Check sheet for the modelled part. Datum: model origin and axes. Units: mm. A direction names the side the tool comes from. Coordinates: 2 decimals unless noted, no trailing zeros. Loops run counter-clockwise (first coordinate to the right, second up) from the corner with the lowest first, then second, coordinate; pieces in that order, holes last. Notation, with made-up numbers: (68.25, 36) -> (121.25, 36) arc R26 ccw to (121.25, 61) -> close; hole circle Ø8 at (4.5, -11). An arc over 180 degrees is marked (long way). Use one line per item in the form item = value.
from build123d import *

# Parameters (mm, degrees)
F0_R     = 10
F1_DEPTH = 1.5
F2_R     = 5
F3_DEPTH = 1
F4_R     = 4
F5_DEPTH = 3
F6_R     = 0.75


with BuildPart() as f1:
    # F0 (on Top) → F1 (new body)
    with BuildSketch(Plane.XY):
        Circle(F0_R)
    extrude(amount=F1_DEPTH)

    # F2 (on face) → F3 (join)
    with BuildSketch(Plane.XY.offset(1.5)):
        Circle(F2_R)
    extrude(amount=F3_DEPTH)

    # F4 (on face) → F5 (join)
    with BuildSketch(Plane.XY.offset(2.5)):
        Circle(F4_R)
    extrude(amount=F5_DEPTH)

    # F6
    f6_edges = [f1.edges().sort_by_distance(p)[0] for p in [
        (-10, 0, 0),
    ]]
    fillet(f6_edges, radius=F6_R)


solid = f1.part
(1) Tool access check on faces 1 (the cylindrical face through (-2.17, -9.76, 1.12)), 2 (the flat face through (-5, -2, 1.5)). Record the directions out of +Z, -Z, +X, -X, +Y, -Y that give a thin tool (end or side, any length) a straight path to the whole face; none if there is none.
Established:
face_1 = +Z, -Z
face_2 = +Z
(2) Section check C-C, the plane z = 1.15. Record the boundary of the cut face in (x, y).
Established:
outline = circle Ø20 at (0, 0)
(3) Section check D-D, the plane z = 2.9. Record the boundary of the cut face in (x, y).
Established:
outline = circle Ø8 at (0, 0)
(4) Section check A-A, the plane x = 0. Record the boundary of the cut face in (y, z).
Established:
outline = (-10, 0.75) arc R0.75 ccw to (-9.25, 0) -> (9.25, 0) arc R0.75 ccw to (10, 0.75) -> (10, 1.5) -> (5, 1.5) -> (5, 2.5) -> (4, 2.5) -> (4, 5.5) -> (-4, 5.5) -> (-4, 2.5) -> (-5, 2.5) -> (-5, 1.5) -> (-10, 1.5) -> close
(5) Go/stop test with flat-tipped pins: P1, Ø2, axis at x = -2.5, z = 2, coming from the -Y side; P2, Ø1.5, axis at y = 4, z = 0.5, coming from the +X side; P3, Ø1, axis at y = 1.5, z = 1, coming from the -X side. Record where each tip stops, or that it passes through.
Established:
P1 = -9.87
P2 = 9.45
P3 = -9.95
(6) Scan lines: line 1 along Z through (x, y) = (4.5, 2.5); line 2 along Z through (x, y) = (0, -4.5); line 3 along Y through (x, z) = (-4, 0.85). Record each from-to range of solid material in increasing order.
Established:
line_1 = 0 to 1.5
line_2 = 0 to 2.5
line_3 = -9.17 to 9.17
